Design review of the part built by this model. Coordinates are the model's own, in mm. A direction names the side the tool comes from. Round coordinates to 2 decimals unless told otherwise and drop trailing zeros. Loops run counter-clockwise (first coordinate to the right, second up) from the corner with the lowest first, then second, coordinate; pieces in that order, holes last. Notation, with made-up numbers: (67, 17.5) -> (84, 17.5) arc R12 ccw to (84, 21.5) -> close; hole circle Ø7 at (-10, 55). An arc over 180 degrees is marked (long way). Answer as CSV lines item,"result". Start each with the question number.
(1) Draft analysis for pull direction X (two halves, no side actions). For faces 1 (the face through (3.7, -3.5, -8.3)), 2 (the face through (3.981, -1.726, -12.916)), 3 (the face through (6.35, 8, 0)), state which applies: +X half, -X half, draft (parallel to the pull), parting line (faces both ways), or undercut.
(2) Take a section at D-D, the plane z = -13.36. Write out the cut boundary in (x, y), and give its area (3 significant figures).
(3) Take a section at B-B, the plane x = 3.75. Write out the cut boundary in (y, z), and give its area (3 significant figures).
(4) To check wall thickness, follow line 1 (Y direction, x = 0.25, z = -0.5). State the ranges of the line that lie inside material, in increasing order. Write a range as from..to.
(5) Machinability: for faces 4 (the face through (3.642, -1.726, 12.468)), 5 (the face through (-3.8, -3.5, -13.4)), which of the approach directions +Z, -Z, +X, -X, +Y, -Y give a long, thin tool a straight path to every point of the face, cutting with its end or side? Answer none if there is none.
(6) Take a section at A-A, the plane z = -8.32. Write out the cut boundary in (x, y).
(7) Take a section at C-C, the plane x = -0.75. Write out the cut boundary in (y, z), and give its area (3 significant figures).
(8) For P1, Ø4, axis at x = -0.5, z = 8.5, coming from the -Y side, flat-tipped, find the tip position at first contact; note if it passes through.
Autodesk Inventor part; units mm, degrees
ref_plane "YZ Plane" through (0, 0, 0) normal (1, 0, 0) x (0, 1, 0)
ref_plane "XZ Plane" through (0, 0, 0) normal (0, 1, 0) x (-1, 0, 0)
ref_plane "XY Plane" through (0, 0, 0) normal (0, 0, 1) x (1, 0, 0)
sketch "Sketch1" plane through (0, 0, 0) normal (0, 1, 0) x (-1, 0, 0)
  line L0 (6.35, 14.5) -> (-6.35, 14.5)
  line L1 (-6.35, 14.5) -> (-6.35, -14.5)
  line L2 (-6.35, -14.5) -> (6.35, -14.5)
  line L3 (6.35, -14.5) -> (6.35, 14.5)
  point P0 (0, 0)
  dimension "d0" = 29
  dimension "d1" = 12.7
  dimension "d2" = 6.35
  dimension "d3" = 14.5
extrude "Extrusion1" add sketch "Sketch1" along normal blind 15.7
sketch "Sketch2" plane through (0, 0, 0) normal (0, -1, 0) x (1, 0, 0)
  line L0 (-6.35, 14.5) -> (6.35, 14.5)
  line L1 (-6.35, -14.5) -> (-6.35, 14.5)
  line L2 (6.35, -14.5) -> (-6.35, -14.5)
  line L3 (6.35, 14.5) -> (6.35, -14.5)
  circle A0 centre (3.75, -13.36) radius 0.5
  circle A1 centre (-3.75, -8.32) radius 0.5
  circle A2 centre (3.75, -8.32) radius 0.5
  circle A3 centre (-3.75, -13.36) radius 0.5
  circle A4 centre (3.75, 11.98) radius 0.5
  circle A5 centre (-3.75, 11.98) radius 0.5
  point P0 (0, 0)
  dimension "d9" = 1
  dimension "d10" = 1
  dimension "d11" = 1
  dimension "d12" = 1
  dimension "d15" = 5.04
  dimension "d17" = 7.5
  dimension "d18" = 3.75
  dimension "d19" = 1
  dimension "d20" = 1
  dimension "d22" = 20.3
  dimension "d28" = 2.52
extrude "Extrusion2" add sketch "Sketch2" along normal blind 3.5 contours A0 | A1 | A2 | A3 | A4 | A5
chamfer "Chamfer2" distance 1.524 angle 45 1 edges at (0, 15.7, -14.5)
equation "\"d10\" = d9"
equation "\"d11\" = d9"
equation "\"d12\" = d9"
equation "\"d19\" = d9"
equation "\"d20\" = d9"
properties part number "RZ03-1A4-D005"
The answers:
1,face 1,"draft"
1,face 2,"undercut"
1,face 3,"+X half"
2,outline,"(-6.35, 0) -> (-4.25, 0) -> (-4.25, -3.5) -> (-3.25, -3.5) -> (-3.25, 0) -> (3.25, 0) -> (3.25, -3.5) -> (4.25, -3.5) -> (4.25, 0) -> (6.35, 0) -> (6.35, 15.32) -> (-6.35, 15.32) -> close"
2,area,"202 mm²"
3,outline,"(-3.5, -13.86) -> (0, -13.86) -> (0, -14.5) -> (14.18, -14.5) -> (15.7, -12.98) -> (15.7, 14.5) -> (0, 14.5) -> (0, 12.48) -> (-3.5, 12.48) -> (-3.5, 11.48) -> (0, 11.48) -> (0, -7.82) -> (-3.5, -7.82) -> (-3.5, -8.82) -> (0, -8.82) -> (0, -12.86) -> (-3.5, -12.86) -> close"
3,area,"465 mm²"
4,line 1,"0..15.7"
5,face 4,"-Y"
5,face 5,"+Z, -Z, +X, -X, -Y"
6,outline,"(-6.35, 0) -> (-4.25, 0) -> (-4.25, -3.5) -> (-3.25, -3.5) -> (-3.25, 0) -> (3.25, 0) -> (3.25, -3.5) -> (4.25, -3.5) -> (4.25, 0) -> (6.35, 0) -> (6.35, 15.7) -> (-6.35, 15.7) -> close"
7,outline,"(0, -14.5) -> (14.18, -14.5) -> (15.7, -12.98) -> (15.7, 14.5) -> (0, 14.5) -> close"
7,area,"454 mm²"
8,P1,"y = 0"
